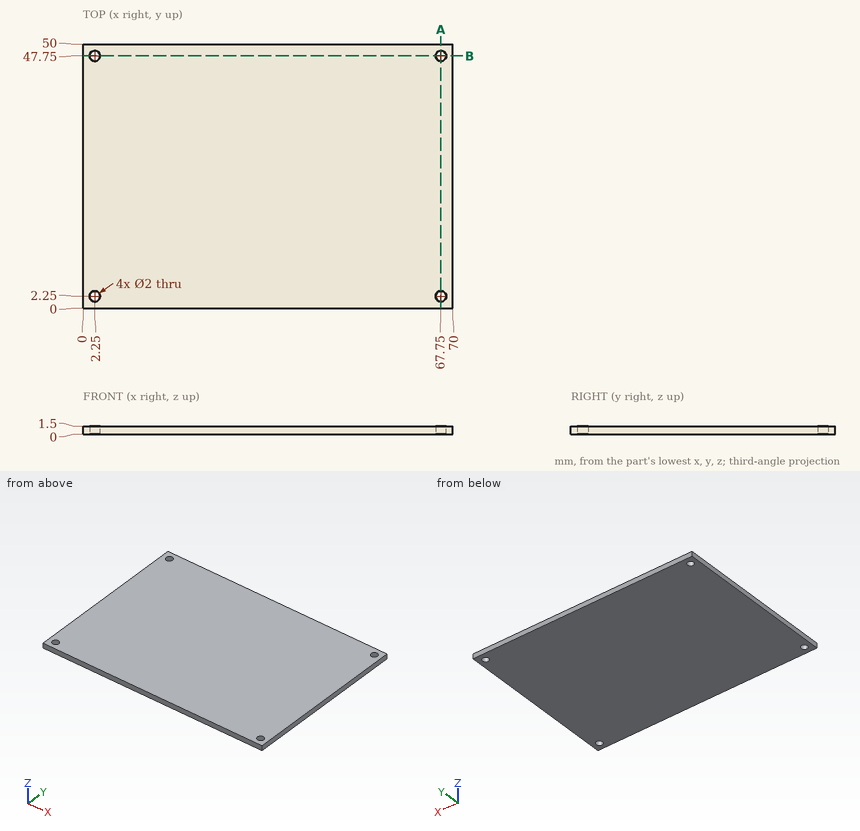
Source: three-view drawing plus pictorial views. Frame: mm from the lowest corner of the part. Round coordinates to 2 decimals unless told otherwise and drop trailing zeros. Loops run counter-clockwise (first coordinate to the right, second up) from the corner with the lowest first, then second, coordinate; pieces in that order, holes last.
Item 1: Line query: L1, parallel to X at y = 47.75, z = 1.05; L2, parallel to Y at x = 67.75, z = 0.65. Output: solid intervals per line, ascending.
Checked values:
L1: x = 0 to 1.25, 3.25 to 66.75, 68.75 to 70
L2: y = 0 to 1.25, 3.25 to 46.75, 48.75 to 50
Item 2: Section B-B, the plane y = 47.75. Output: boundary loops of the cut face in (x, z), plus the area to 3 significant figures.
Checked values:
outline: (0, 0) - (1.25, 0) - (1.25, 1.5) - (0, 1.5) - close; (3.25, 0) - (66.75, 0) - (66.75, 1.5) - (3.25, 1.5) - close; (68.75, 0) - (70, 0) - (70, 1.5) - (68.75, 1.5) - close
area: 99.0 mm2
Item 3: Section A-A, the plane x = 67.75. Output: boundary loops of the cut face in (y, z), plus the area to 3 significant figures.
Checked values:
outline: (0, 0) - (1.25, 0) - (1.25, 1.5) - (0, 1.5) - close; (3.25, 0) - (46.75, 0) - (46.75, 1.5) - (3.25, 1.5) - close; (48.75, 0) - (50, 0) - (50, 1.5) - (48.75, 1.5) - close
area: 69.0 mm2
